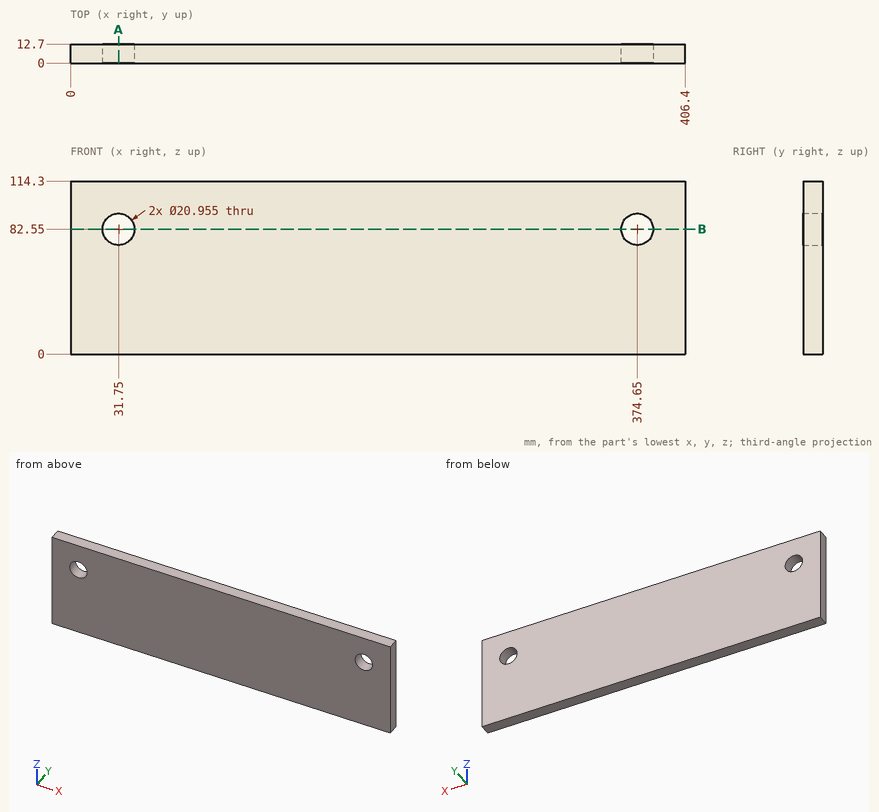
Answer from the drawing. Dimensions are ordinates in mm from the lowest x, y and z of the part. Round coordinates to 2 decimals unless told otherwise and drop trailing zeros. Loops run counter-clockwise (first coordinate to the right, second up) from the corner with the lowest first, then second, coordinate; pieces in that order, holes last.
Q1. Consider probe 1 along X at (y, z) = (10, 82.55); probe 2 along Z at (x, y) = (374.65, 9.75). Determine where each line is inside the solid, lowest interval first.
Q2. Section A-A on x = 31.75 is taken. Write down the section's boundary in (y, z), and give its area (3 significant figures).
Q3. Section B-B on z = 82.55 is taken. Write down the section's boundary in (x, y).
Output:
1. probe 1: x = 0 to 21.27, 42.23 to 364.17, 385.13 to 406.4
1. probe 2: z = 0 to 72.07, 93.03 to 114.3
2. outline: (0, 0) - (12.7, 0) - (12.7, 72.07) - (0, 72.07) - close; (0, 93.03) - (12.7, 93.03) - (12.7, 114.3) - (0, 114.3) - close
2. area: 1,190 mm2
3. outline: (0, 0) - (21.27, 0) - (21.27, 12.7) - (0, 12.7) - close; (42.23, 0) - (364.17, 0) - (364.17, 12.7) - (42.23, 12.7) - close; (385.13, 0) - (406.4, 0) - (406.4, 12.7) - (385.13, 12.7) - close
